Read the model definition and answer for the solid it produces. Units are mm, in the model's axes. A direction names the side the tool comes from. Round coordinates to 2 decimals unless told otherwise and drop trailing zeros. Write each loop counter-clockwise with the first axis right and the second up, starting at its lowest first coordinate (ties: lowest second). Pieces come first, ordered by that corner, then holes. Notation, with made-up numbers: (8.25, 28.5) - (64.25, 28.5) arc R36 cw to (64.25, 66.5) - close; hole circle Ø3 at (10.5, 47). An arc over 180 degrees is marked (long way). One line per item, written item: value. Start each with the question number.
(1) Find the intervals of material crossed by L1, parallel to Z at x = 2.75, y = -0.55; L2, parallel to X at y = -1.9, z = -5; L3, parallel to Z at x = -1, y = 0.95, in increasing order.
(2) The mould has two halves that part along Z. Classify faces 5 (the face through (0, 0, -10)), 6 (the face through (0.71, 1.64, -4.46)), 7 (the face through (-0.596, -2.685, -10.493)): +Z half, -Z half, draft (parallel to the pull), parting line (faces both ways), or undercut.
(3) A cutting plane is placed at B-B, the plane y = -1.5. Determine the outline of the cut face in (x, z), plus the area to 3 significant figures.
(4) A cutting plane is placed at C-C, the plane z = -44.5. Determine the outline of the cut face in (x, y), plus the area to 3 significant figures.
(5) A cutting plane is placed at A-A, the plane z = -5. Determine the outline of the cut face in (x, y).
(6) Flat-ended cylindrical pins translate along their axes: pin 1 Ø2 at (y, z) = (0.5, -7) entering from +X; pin 2 Ø1 at (x, z) = (1.5, -18.5) entering from -Y; pin 3 Ø3 at (x, z) = (-0.13, -5) entering from +Y. Find the tip coordinate at first contact, or state that the pin passes through.
(7) For faces 1 (the face through (-0.54, -2.44, -33.14)), 2 (the face through (0, 2.5, -3.8)), 3 (the face through (1.02, 0.8, -4.93)), 4 (the face through (0, -2.5, -3.8)), determine the directions among +Z, -Z, +X, -X, +Y, -Y from which every point of the face is accessible in a straight line to the end or side of a thin tool.
from build123d import *

# Parameters (mm, degrees)
SKETCH1_R               = 2.5
BOSS_EXTRUDE1_DEPTH     = 59.4
CUT_EXTRUDE1_DEPTH      = 10
SKETCH3_R               = 2.75
BOSS_EXTRUDE2_DEPTH     = 1
FILLET1_R               = 2.5
BOSS_EXTRUDE3_DEPTH     = 1
CUT_EXTRUDE2_DEPTH      = 60.549382271
CUT_EXTRUDE2_DEPTH_BACK = 60.549382271
SKETCH5_R               = 1


with BuildPart() as part:
    # Sketch1 → Boss-Extrude1 (new body)
    with BuildSketch(Plane.XY):
        Circle(SKETCH1_R)
    extrude(amount=-BOSS_EXTRUDE1_DEPTH)

    # Sketch2 → Cut-Extrude1 (cut)
    with BuildSketch(Plane.XY):
        with BuildLine():
            Line((-2.368543856, 0.8), (2.368543856, 0.8))
            ThreePointArc((2.368543856, 0.8), (2.5, 0), (2.368543856, -0.8))
            Line((2.368543856, -0.8), (-2.368543856, -0.8))
            ThreePointArc((-2.368543856, -0.8), (-2.5, 0), (-2.368543856, 0.8))
        make_face()
    extrude(amount=-CUT_EXTRUDE1_DEPTH, mode=Mode.SUBTRACT)

    # Sketch3 → Boss-Extrude2 (add)
    with BuildSketch(Plane.XY.offset(-10)):
        Circle(SKETCH3_R)
    extrude(amount=-BOSS_EXTRUDE2_DEPTH)

    # Fillet1
    fillet1_edges = [part.edges().sort_by_distance(p)[0] for p in [
        (-2.5, 0, -59.4),
    ]]
    fillet(fillet1_edges, radius=FILLET1_R)

    # Sketch4 → Boss-Extrude3 (add)
    with BuildSketch(Plane.XY.offset(-56.9)):
        Polygon((1.547782106, 2.772670894), (-1.627312377, 2.726754071), (-3.175094483, -0.045916823), (-1.547782106, -2.772670894), (1.627312377, -2.726754071), (3.175094483, 0.045916823), align=None)
    extrude(amount=BOSS_EXTRUDE3_DEPTH)

    # Sketch5 → Cut-Extrude2 (cut, two sides: drawn at the far end of the back side and taken through both)
    with BuildSketch(Plane(origin=(0, 0, 0), x_dir=(1, 0, 0), z_dir=(0, 1, 0)).offset(-CUT_EXTRUDE2_DEPTH_BACK)):
        with Locations(Location((-0.131456144, 5, 0), (0, 0, 270))):
            Circle(SKETCH5_R)
    extrude(amount=CUT_EXTRUDE2_DEPTH + CUT_EXTRUDE2_DEPTH_BACK, mode=Mode.SUBTRACT)


solid = part.part
Here are the results:
1. L1: -56.9 to -55.9
1. L2: -1.62 to -1.13, 0.87 to 1.62
1. L3: -58.99 to -5.5, -4.5 to 0
2. face 5: +Z half
2. face 6: undercut
2. face 7: draft
3. outline: (-2.31, -56.9) - (-2, -56.9) arc R2 ccw to (2, -56.9) - (2.31, -56.9) - (2.31, -55.9) - (2, -55.9) - (2, -11) - (2.3, -11) - (2.3, -10) - (2, -10) - (2, 0) - (-2, 0) - (-2, -10) - (-2.3, -10) - (-2.3, -11) - (-2, -11) - (-2, -55.9) - (-2.31, -55.9) - close; hole circle Ø2 at (-0.13, -5)
3. area: 232 mm²
4. outline: circle Ø5 at (0, 0)
4. area: 19.6 mm²
5. outline: (-2.37, -0.8) arc R2.5 ccw to (-1.13, -2.23) - (-1.13, -0.8) - close; (-2.37, 0.8) - (-1.13, 0.8) - (-1.13, 2.23) arc R2.5 ccw to start; (0.87, -2.34) arc R2.5 ccw to (2.37, -0.8) - (0.87, -0.8) - close; (0.87, 0.8) - (2.37, 0.8) arc R2.5 ccw to (0.87, 2.34) - close
6. pin 1: x = 2.37
6. pin 2: y = -2.29
6. pin 3: y = 2.5
7. face 1: none
7. face 2: +Z, +Y
7. face 3: +Z, +X, -X
7. face 4: +Z, -Y
